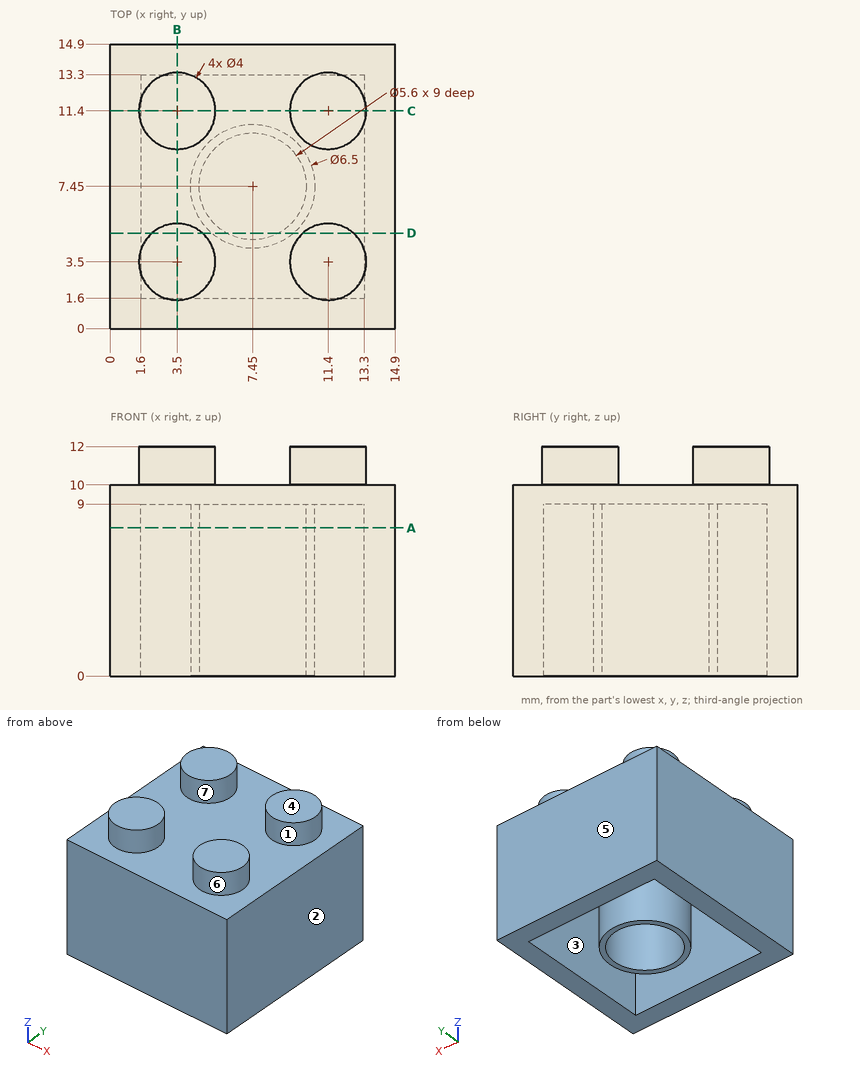
Print and shaded views of the part. All mm, measured from the part's lowest x, y and z. A direction names the side the tool comes from. Give positions to 0.01 mm unless a question says otherwise; leave off trailing zeros. Loops run counter-clockwise (first coordinate to the right, second up) from the corner with the lowest first, then second, coordinate; pieces in that order, holes last. Notation, with made-up numbers: (-26, 33) - (-14, 33) arc R9 cw to (-14, 46) - close; hole circle Ø8 at (60.5, 54). An arc over 180 degrees is marked (long way). One line per item, written item: value. Start each with the question number.
1. Which spindle directions (+Z, -Z, +X, -X, +Y, -Y) get a long thin tool onto all of the face, cutting with end or side? Do the marked faces 1, 2 and 3. Say none if no direction does.
2. Slice it at B-B (x = 3.5). List the corners of the cut face in (y, z), plus the area to 3 significant figures.
3. Slice it at A-A (z = 7.75). List the corners of the cut face in (x, y).
4. Pull direction Y, two halves, no side cores. Call the marked faces 4, 5, 6 and 7: pulls with the +Y half, pulls with the -Y half, needs draft (parallel to the pull), parting line crosses it, or undercut.
5. Slice it at D-D (y = 5). List the corners of the cut face in (x, z), plus the area to 3 significant figures.
6. Pin check, flat tip, straight feed: pin 1 (3.5 mm diameter, centred on x = 7.45, y = 7.45, fed in from -Z). Stop position of the tip, or through.
7. Probe L1, parallel to Y at x = 7.45, z = 3.75; L2, parallel to X at y = 1.75, z = 4.5. List the from-to ranges inside material, lowest first. Write a range as from..to.
Solution:
1. face 1: +Z
1. face 2: +Z, -Z, +X, +Y, -Y
1. face 3: -Z
2. outline: (0, 0) - (1.6, 0) - (1.6, 9) - (13.3, 9) - (13.3, 0) - (14.9, 0) - (14.9, 10) - (13.4, 10) - (13.4, 12) - (9.4, 12) - (9.4, 10) - (5.5, 10) - (5.5, 12) - (1.5, 12) - (1.5, 10) - (0, 10) - close
2. area: 59.7 mm^2
3. outline: (0, 0) - (14.9, 0) - (14.9, 14.9) - (0, 14.9) - close; circle Ø6.5 at (7.45, 7.45); hole (1.6, 1.6) - (13.3, 1.6) - (13.3, 13.3) - (1.6, 13.3) - close; hole circle Ø5.6 at (7.45, 7.45)
4. face 4: needs draft
4. face 5: pulls with the +Y half
4. face 6: undercut
4. face 7: undercut
5. outline: (0, 0) - (1.6, 0) - (1.6, 9) - (5.31, 9) - (5.31, 0) - (6.09, 0) - (6.09, 9) - (8.81, 9) - (8.81, 0) - (9.59, 0) - (9.59, 9) - (13.3, 9) - (13.3, 0) - (14.9, 0) - (14.9, 10) - (12.72, 10) - (12.72, 12) - (10.08, 12) - (10.08, 10) - (4.82, 10) - (4.82, 12) - (2.18, 12) - (2.18, 10) - (0, 10) - close
5. area: 68.3 mm^2
6. pin 1: stops at z = 9
7. L1: y = 0..1.6, 4.2..4.65, 10.25..10.7, 13.3..14.9
7. L2: x = 0..1.6, 13.3..14.9
